```python
from build123d import *

# Parameters (mm, degrees)
SKETCH1_W                      = 18
SKETCH1_H                      = 25.4
SKETCH1_R                      = 0.9
BOSS_EXTRUDE1_DEPTH            = 20
CBORE_FOR_M5_SHCS1_D           = 5.5
CBORE_FOR_M5_SHCS1_CBORE_D     = 10
CBORE_FOR_M5_SHCS1_CBORE_DEPTH = 12
FILLET1_R                      = 10


with BuildPart() as part:
    # Sketch1 → Boss-Extrude1 (new body)
    with BuildSketch(Plane(origin=(0, 0, 0), x_dir=(1, 0, 0), z_dir=(0, 1, 0))):
        Rectangle(SKETCH1_W, SKETCH1_H)
        with Locations(Location((-6.25, 10.6299, 0), (0, 0, 270))):
            Circle(SKETCH1_R, mode=Mode.SUBTRACT)
        with Locations(Location((6.25, 10.6299, 0), (0, 0, 270))):
            Circle(SKETCH1_R, mode=Mode.SUBTRACT)
        with Locations(Location((6.25, -10.6299, 0), (0, 0, 270))):
            Circle(SKETCH1_R, mode=Mode.SUBTRACT)
        with Locations(Location((-6.25, -10.6299, 0), (0, 0, 270))):
            Circle(SKETCH1_R, mode=Mode.SUBTRACT)
    extrude(amount=BOSS_EXTRUDE1_DEPTH)

    # CBORE for M5 SHCS1 (through all)
    with Locations(Plane(origin=(9, 0, 0), x_dir=(0, 0, -1), z_dir=(1, 0, 0))):
        with Locations((-5.7, 10), (5.7, 10)):
            CounterBoreHole(CBORE_FOR_M5_SHCS1_D / 2, CBORE_FOR_M5_SHCS1_CBORE_D / 2, CBORE_FOR_M5_SHCS1_CBORE_DEPTH)

    # Fillet1
    # the kernel refuses this fillet: 10 mm, written as the material it takes off along each edge
    with BuildSketch(Plane(origin=(9, 0, -37.7), x_dir=(0, 1, 0), z_dir=(0, 0, 1))) as fillet1_piece_1:
        with BuildLine():
            CenterArc((FILLET1_R, FILLET1_R), FILLET1_R, 180, 90)
            Line((0, FILLET1_R), (0, 0))
            Line((0, 0), (FILLET1_R, 0))
        make_face()
    extrude(amount=75.4, mode=Mode.SUBTRACT)


solid = part.part
```
Input: part model. Units: mm. Frame: model coordinates. A direction names the side the tool comes from. Give positions to 0.01 mm unless a question says otherwise; leave off trailing zeros. Loops run counter-clockwise (first coordinate to the right, second up) from the corner with the lowest first, then second, coordinate; pieces in that order, holes last. Notation, with made-up numbers: M 89,10.25 L 126,10.25 A26 ccw 126,43.25 Z; hole C 42,64.5 d5. An arc over 180 degrees is marked long. Answer as CSV lines item,"result". Start each with the question number.
1. Reachability of faces 4 (the face through (-3, 8, -8)), 5 (the face through (5.905, 11.011, 11.461)) from +Z, -Z, +X, -X, +Y, -Y: full face, straight path, thin tool, end or side. Return the list, or none.
2. Pin query (flat end, axial travel): P1, Ø6, axis at y = 10, z = -5.7, coming from the +X side; P2, Ø4.5, axis at y = 10, z = 5.7, coming from the +X side; P3, Ø2.5, axis at x = 6.25, z = -10.63, coming from the -Y side; P4, Ø1.5, axis at x = 7, z = 4.5, coming from the -Y side. Return the tip coordinate at first contact, or that it passes through.
3. Pull-direction query (Y, two-part tool) for faces 1 (the face through (-5, 0, 0)), 2 (the face through (-9, 10, 0)), 3 (the face through (-3, 7.8, 3.5)); classes: released by +Y, released by -Y, zero draft, split by the parting line, or undercut.
4. Section C-C on z = 5.7. Return loops of the section in (x, y).
5. Section B-B on y = 16.5. Return loops of the section in (x, z), plus the area to 3 significant figures.
6. Section D-D on x = -2. Return loops of the section in (y, z), plus the area to 3 significant figures.
7. Line query: L1, parallel to Z at x = 6.25, y = 18.5; L2, parallel to Z at x = 5.25, y = 7.5; L3, parallel to X at y = 10, z = -2. Output: solid intervals per line, ascending.
8. Section A-A on x = -6.25. Return loops of the section in (y, z).
Computed values:
1,face 4,"+X"
1,face 5,"+Y, -Y"
2,P1,"stops at x = -3"
2,P2,"passes through"
2,P3,"stops at y = 2"
2,P4,"stops at y = 3.11"
3,face 1,"released by -Y"
3,face 2,"zero draft"
3,face 3,"undercut"
4,outline,"M -9,0 L -1,0 A10 ccw 7.66,5 L -3,5 L -3,7.25 L -9,7.25 Z; M -9,12.75 L -3,12.75 L -3,15 L 9,15 L 9,20 L -9,20 Z"
5,outline,"M -9,-12.7 L 9,-12.7 L 9,12.7 L -9,12.7 Z; hole C -6.25,-10.63 d1.8; hole C -6.25,10.63 d1.8; hole C 6.25,-10.63 d1.8; hole C 6.25,10.63 d1.8"
5,area,"447 mm²"
6,outline,"M 0,-12.7 L 20,-12.7 L 20,12.7 L 0,12.7 Z; hole C 10,-5.7 d10; hole C 10,5.7 d10"
6,area,"351 mm²"
7,L1,"z = -12.7 to -11.53, -9.73 to 9.73, 11.53 to 12.7"
7,L2,"z = -12.7 to -10.03, -1.37 to 1.37, 10.03 to 12.7"
7,L3,"x = -9 to -3"
8,outline,"M 0,-12.7 L 20,-12.7 L 20,-11.53 L 0,-11.53 Z; M 0,-9.73 L 20,-9.73 L 20,9.73 L 0,9.73 Z; M 0,11.53 L 20,11.53 L 20,12.7 L 0,12.7 Z; hole C 10,-5.7 d5.5; hole C 10,5.7 d5.5"
